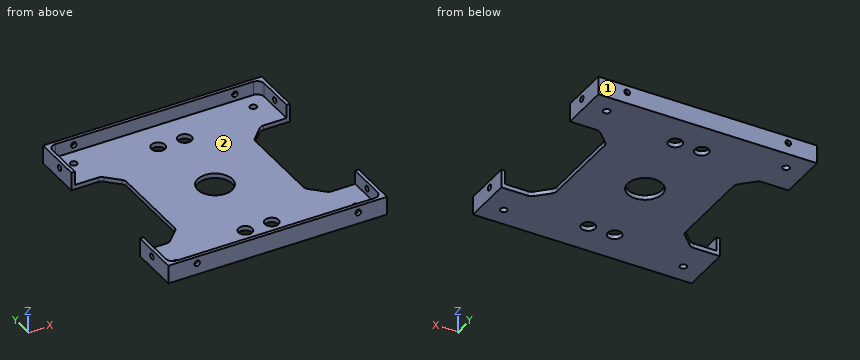
from build123d import *

# Parameters (mm, degrees)
SKETCH1_W                       = 96
SKETCH1_H                       = 96
BOSS_EXTRUDE1_DEPTH             = 8
SKETCH2_W                       = 92
SKETCH2_H                       = 92
COMPONENT_PLATFORM_DEPTH        = 6
CABLE_SLOTS_DEPTH               = 6
SKETCH4_R                       = 7.5
CENTER_MASS_CUT_DEPTH           = 6
INNER_CORNER_FILLETS_R          = 3
TAP_DRILL_FOR_M3X0_5_TAP1_D     = 2.5
TAP_DRILL_FOR_M3X0_5_TAP1_DEPTH = 2
TAP_DRILL_FOR_M3X0_5_TAP2_D     = 2.5
TAP_DRILL_FOR_M3X0_5_TAP2_DEPTH = 2
F_3_0MM_DOWEL_HOLE3_D           = 3
F_3_0MM_DOWEL_HOLE3_DEPTH       = 10
F_3_0MM_DOWEL_HOLE3_TIP         = 0.901290929
CUT_EXTRUDE1_START              = -8
SKETCH16_OUTSIDE_W              = 125.2
SKETCH16_OUTSIDE_H              = 125.2
SKETCH16_OUTSIDE_W_2            = 95
SKETCH16_OUTSIDE_H_2            = 95
CUT_EXTRUDE1_DEPTH              = 8
SKETCH17_R                      = 3
CUT_EXTRUDE3_DEPTH              = 9


with BuildPart() as part:
    # Sketch1 → Boss-Extrude1 (new body)
    with BuildSketch(Plane.XY):
        Rectangle(SKETCH1_W, SKETCH1_H)
    extrude(amount=BOSS_EXTRUDE1_DEPTH)

    # Sketch2 → Component Platform (cut)
    with BuildSketch(Plane.XY.offset(8)):
        Rectangle(SKETCH2_W, SKETCH2_H)
    extrude(amount=-COMPONENT_PLATFORM_DEPTH, mode=Mode.SUBTRACT)

    # Sketch3 → Cable Slots (cut, symmetric)
    with BuildSketch(Plane.XY.offset(2)):
        with BuildLine():
            Line((-33.878679656, -25.121320344), (-28.878679656, -20.121320344))
            ThreePointArc((-28.878679656, -20.121320344), (-28.228361402, -19.148050297), (-28, -18))
            Line((-28, -18), (-28, 18))
            ThreePointArc((-28, 18), (-28.228361402, 19.148050297), (-28.878679656, 20.121320344))
            Line((-28.878679656, 20.121320344), (-33.878679656, 25.121320344))
            ThreePointArc((-33.878679656, 25.121320344), (-34.851949703, 25.771638598), (-36, 26))
            Line((-36, 26), (-48, 26))
            Line((-48, 26), (-48, -26))
            Line((-48, -26), (-36, -26))
            ThreePointArc((-36, -26), (-34.851949703, -25.771638598), (-33.878679656, -25.121320344))
        make_face()
        with BuildLine():
            Line((48, -26), (48, 26))
            Line((48, 26), (36, 26))
            ThreePointArc((36, 26), (34.851949703, 25.771638598), (33.878679656, 25.121320344))
            Line((33.878679656, 25.121320344), (28.878679656, 20.121320344))
            ThreePointArc((28.878679656, 20.121320344), (28.228361402, 19.148050297), (28, 18))
            Line((28, 18), (28, -18))
            ThreePointArc((28, -18), (28.228361402, -19.148050297), (28.878679656, -20.121320344))
            Line((28.878679656, -20.121320344), (33.878679656, -25.121320344))
            ThreePointArc((33.878679656, -25.121320344), (34.851949703, -25.771638598), (36, -26))
            Line((36, -26), (48, -26))
        make_face()
    extrude(amount=CABLE_SLOTS_DEPTH, both=True, mode=Mode.SUBTRACT)

    # Sketch4 → Center Mass Cut (cut)
    with BuildSketch(Plane.XY.offset(2)):
        Circle(SKETCH4_R)
    extrude(amount=-CENTER_MASS_CUT_DEPTH, mode=Mode.SUBTRACT)

    # Inner Corner Fillets
    inner_corner_fillets_edges = [part.edges().sort_by_distance(p)[0] for p in [
        (-46, -46, 5),
        (-46, 46, 5),
        (46, 46, 5),
        (46, -46, 5),
    ]]
    fillet(inner_corner_fillets_edges, radius=INNER_CORNER_FILLETS_R)

    # Tap Drill for M3x0.5 Tap1
    with Locations(Plane(origin=(0, -48, 0), x_dir=(-1, 0, 0), z_dir=(0, -1, 0))):
        with Locations((35, -5), (-35, -5)):
            tap_drill_for_m3x0_5_tap1 = Hole(TAP_DRILL_FOR_M3X0_5_TAP1_D / 2, depth=TAP_DRILL_FOR_M3X0_5_TAP1_DEPTH)

    # Tap Drill for M3x0.5 Tap2
    with Locations(Plane(origin=(48, 0, 0), x_dir=(0, 0, -1), z_dir=(1, 0, 0))):
        with Locations((-5, -35), (-5, 35)):
            tap_drill_for_m3x0_5_tap2 = Hole(TAP_DRILL_FOR_M3X0_5_TAP2_D / 2, depth=TAP_DRILL_FOR_M3X0_5_TAP2_DEPTH)

    # Mirror1: Tap Drill for M3x0.5 Tap1 across plane
    add(tap_drill_for_m3x0_5_tap1.mirror(Plane(origin=(0, 0, 0), x_dir=(0, 0, 1), z_dir=(0, -1, 0))), mode=Mode.SUBTRACT)

    # Mirror2: Tap Drill for M3x0.5 Tap2 across plane
    add(tap_drill_for_m3x0_5_tap2.mirror(Plane(origin=(0, 0, 0), x_dir=(0, 0, 1), z_dir=(1, 0, 0))), mode=Mode.SUBTRACT)

    # Ø3.0mm Dowel Hole3
    with Locations(Plane.XY.offset(2)):
        with Locations((-39, -39), (39, -39), (39, 39), (-39, 39)):
            Hole(F_3_0MM_DOWEL_HOLE3_D / 2, depth=F_3_0MM_DOWEL_HOLE3_DEPTH)
            with Locations((0, 0, -(F_3_0MM_DOWEL_HOLE3_DEPTH + F_3_0MM_DOWEL_HOLE3_TIP / 2))):  # 118° drill point
                Cone(0, F_3_0MM_DOWEL_HOLE3_D / 2, F_3_0MM_DOWEL_HOLE3_TIP, mode=Mode.SUBTRACT)

    # Sketch16 outside → Cut-Extrude1 (cut)
    with BuildSketch(Plane(origin=(0, 0, 0), x_dir=(-1, 0, 0), z_dir=(0, 0, -1)).offset(CUT_EXTRUDE1_START)):
        Rectangle(SKETCH16_OUTSIDE_W, SKETCH16_OUTSIDE_H)
        Rectangle(SKETCH16_OUTSIDE_W_2, SKETCH16_OUTSIDE_H_2, mode=Mode.SUBTRACT)
    extrude(amount=CUT_EXTRUDE1_DEPTH, mode=Mode.SUBTRACT)

    # Sketch17 → Cut-Extrude3 (cut, through all)
    with BuildSketch(Plane(origin=(0, 0, 0), x_dir=(-1, 0, 0), z_dir=(0, 0, -1))):
        with Locations((-5.755, -32.99999626)):
            Circle(SKETCH17_R)
        with Locations((5.755, -32.99999626)):
            Circle(SKETCH17_R)
    cut_extrude3 = extrude(amount=-CUT_EXTRUDE3_DEPTH, mode=Mode.SUBTRACT)

    # Mirror4: Cut-Extrude3 across plane
    add(cut_extrude3.mirror(Plane(origin=(0, 0, 0), x_dir=(0, 0, 1), z_dir=(0, -1, 0))), mode=Mode.SUBTRACT)


solid = part.part
For this review, take the finished solid that the model builds, in its own axes (mm). Face numbers are marked on the shaded views. Round coordinates to 2 decimals unless told otherwise and drop trailing zeros. Order: outer loops, then holes, each group sorted by start corner. A loop starts at its lowest first (then second) coordinate and runs counter-clockwise, first axis right, second up. Notation, with made-up numbers: (-34, -33) -> (-15, -33) arc R21 ccw to (-15, -16) -> close; hole circle Ø11 at (77, 8.5). An arc over 180 degrees is marked (long way). Write item = value, one per line. Start each with the question number.
1) To check wall thickness, follow line 1 (Y direction, x = 39, z = 1.2); line 2 (Y direction, x = -27, z = 7.5); line 3 (X direction, y = -46.4, z = 5). State the ranges of each line that lie inside material, in increasing order. Write a range as from..to.
2) The part is to be moulded in two halves that separate along X. For the marked faces 1 and 2, say which applies: +X half, -X half, draft (parallel to the pull), parting line (faces both ways), or undercut.
3) Take a section at A-A on y = 0. State the section outline as (x, z) points.
4) Take a section at C-C on x = 10. State the section outline as (y, z) points, plus the area to 3 significant figures.
5) Insertion check: pin 1 (4 mm diameter, centred on x = -39, y = 39, fed in from +Z); pin 2 (1 mm diameter, centred on y = 5, z = 1.5, fed in from +X); pin 3 (2 mm diameter, centred on x = 35, z = 5, fed in from -Y). Each pin has a flat end and moves straight along its axis. Give the tip position at first contact, or say it passes through.
6) Take a section at B-B on y = -39. State the section outline as (x, z) points.
7) Take a section at D-D on x = -0.5. State the section outline as (y, z) points.
Verdict:
q1.line_1 = -47.5..-40.5, -37.5..-26, 26..37.5, 40.5..47.5
q1.line_2 = -47.5..-46, 46..47.5
q1.line_3 = -47.5..-36.25, -33.75..33.75, 36.25..47.5
q2.face_1 = draft
q2.face_2 = undercut
q3.outline = (-28, 0) -> (-7.5, 0) -> (-7.5, 2) -> (-28, 2) -> close; (7.5, 0) -> (28, 0) -> (28, 2) -> (7.5, 2) -> close
q4.outline = (-47.5, 0) -> (47.5, 0) -> (47.5, 8) -> (46, 8) -> (46, 2) -> (-46, 2) -> (-46, 8) -> (-47.5, 8) -> close
q4.area = 208 mm2
q5.pin_1 = 2
q5.pin_2 = 28
q5.pin_3 = through
q6.outline = (-47.5, 0) -> (-40.5, 0) -> (-40.5, 2) -> (-46, 2) -> (-46, 8) -> (-47.5, 8) -> close; (-37.5, 0) -> (37.5, 0) -> (37.5, 2) -> (-37.5, 2) -> close; (40.5, 0) -> (47.5, 0) -> (47.5, 8) -> (46, 8) -> (46, 2) -> (40.5, 2) -> close
q7.outline = (-47.5, 0) -> (-7.48, 0) -> (-7.48, 2) -> (-46, 2) -> (-46, 8) -> (-47.5, 8) -> close; (7.48, 0) -> (47.5, 0) -> (47.5, 8) -> (46, 8) -> (46, 2) -> (7.48, 2) -> close
